from build123d import *

# Parameters (mm, degrees)
SKETCH1_W               = 673.1
SKETCH1_H               = 152.4
BOSS_EXTRUDE1_DEPTH     = 7.9375
SKETCH2_W               = 7.9375
SKETCH2_H               = 123.825
SKETCH2_W_2             = 644.525
SKETCH2_H_2             = 7.9375
BOSS_EXTRUDE2_DEPTH     = 15.875
FILLET1_R               = 6.35
SKETCH3_R               = 9.525
SKETCH3_R_2             = 6.35
CUT_EXTRUDE1_DEPTH      = 1
CUT_EXTRUDE1_DEPTH_BACK = 16.875


with BuildPart() as part:
    # Sketch1 → Boss-Extrude1 (new body, symmetric)
    with BuildSketch(Plane.XY):
        Rectangle(SKETCH1_W, SKETCH1_H)
    extrude(amount=BOSS_EXTRUDE1_DEPTH, both=True)

    # Sketch2 → Boss-Extrude2 (add)
    with BuildSketch(Plane.XY.offset(7.9375)):
        with Locations((-340.51875, 0)):
            Rectangle(SKETCH2_W, SKETCH2_H)
        with Locations((0, 80.16875)):
            Rectangle(SKETCH2_W_2, SKETCH2_H_2)
        with Locations((0, -80.16875)):
            Rectangle(SKETCH2_W_2, SKETCH2_H_2)
        with Locations((340.51875, 0)):
            Rectangle(SKETCH2_W, SKETCH2_H)
    extrude(amount=-BOSS_EXTRUDE2_DEPTH)

    # Fillet1
    fillet1_edges = [part.edges().sort_by_distance(p)[0] for p in [
        (-336.55, -61.9125, 0),
        (-336.55, 61.9125, 0),
        (322.2625, 76.2, 0),
        (-322.2625, 76.2, 0),
        (322.2625, -76.2, 0),
        (-322.2625, -76.2, 0),
        (336.55, 61.9125, 0),
        (336.55, -61.9125, 0),
    ]]
    fillet(fillet1_edges, radius=FILLET1_R)

    # Sketch3 → Cut-Extrude1 (cut, two sides)
    with BuildSketch(Plane.XY.offset(7.9375)) as cut_extrude1_sk:
        with Locations((0, -60.325)):
            Circle(SKETCH3_R)
        with Locations((0, 63.5)):
            Circle(SKETCH3_R_2)
        with Locations((25.4, 63.5)):
            Circle(SKETCH3_R_2)
        with Locations((50.8, 63.5)):
            Circle(SKETCH3_R_2)
        with Locations((76.2, 63.5)):
            Circle(SKETCH3_R_2)
        with Locations((101.6, 63.5)):
            Circle(SKETCH3_R_2)
        with Locations((127, 63.5)):
            Circle(SKETCH3_R_2)
        with Locations((152.4, 63.5)):
            Circle(SKETCH3_R_2)
        with Locations((177.8, 63.5)):
            Circle(SKETCH3_R_2)
        with Locations((203.2, 63.5)):
            Circle(SKETCH3_R_2)
        with Locations((228.6, 63.5)):
            Circle(SKETCH3_R_2)
        with Locations((254, 63.5)):
            Circle(SKETCH3_R_2)
        with Locations((279.4, 63.5)):
            Circle(SKETCH3_R_2)
        with Locations((304.8, 63.5)):
            Circle(SKETCH3_R_2)
        with Locations((-25.4, 63.5)):
            Circle(SKETCH3_R_2)
        with Locations((-50.8, 63.5)):
            Circle(SKETCH3_R_2)
        with Locations((-76.2, 63.5)):
            Circle(SKETCH3_R_2)
        with Locations((-101.6, 63.5)):
            Circle(SKETCH3_R_2)
        with Locations((-127, 63.5)):
            Circle(SKETCH3_R_2)
        with Locations((-152.4, 63.5)):
            Circle(SKETCH3_R_2)
        with Locations((-177.8, 63.5)):
            Circle(SKETCH3_R_2)
        with Locations((-203.2, 63.5)):
            Circle(SKETCH3_R_2)
        with Locations((-228.6, 63.5)):
            Circle(SKETCH3_R_2)
        with Locations((-254, 63.5)):
            Circle(SKETCH3_R_2)
        with Locations((-279.4, 63.5)):
            Circle(SKETCH3_R_2)
        with Locations((-304.8, 63.5)):
            Circle(SKETCH3_R_2)
        with Locations((293.6875, -60.325)):
            Circle(SKETCH3_R)
        with Locations((-293.6875, -60.325)):
            Circle(SKETCH3_R)
    extrude(amount=CUT_EXTRUDE1_DEPTH, mode=Mode.SUBTRACT)
    extrude(cut_extrude1_sk.sketch, amount=-CUT_EXTRUDE1_DEPTH_BACK, mode=Mode.SUBTRACT)


solid = part.part
Source: CAD feature listing. Evaluate the final solid. Frame: model axes, mm. Give positions to 0.01 mm unless a question says otherwise; leave off trailing zeros. Write each loop counter-clockwise with the first axis right and the second up, starting at its lowest first coordinate (ties: lowest second). Pieces come first, ordered by that corner, then holes. Notation, with made-up numbers: M 46,18.25 L 66,18.25 A22 cw 66,48.25 Z; hole C 16,-38.75 d7. An arc over 180 degrees is marked long. Answer as a JSON object with one key per item and string values.
Q1. Ray query, line 1 along X through (y, z) = (-59, -6.5); line 2 along Y through (x, z) = (151.5, -0.75); line 3 along X through (y, z) = (-71, 2.75). Return the intervals inside material, ascending.
Geometry check:
{"line 1": "x = -344.49 to -303.12, -284.26 to -9.43, 9.43 to 284.26, 303.12 to 344.49", "line 2": "y = -84.14 to 57.21, 69.79 to 84.14", "line 3": "x = -336.55 to 336.55"}
Q2. Mould query, pull axis X, two halves, no side actions, for faces 1 (the face through (-26.78, 57.3, 0.11)), 2 (the face through (302.486, -63.973, 0.111)), 3 (the face through (-344.488, -1, 0)), 4 (the face through (-5, 84.138, 0)). Classes: +X half, -X half, draft (parallel to the pull), parting line (faces both ways), or undercut.
Geometry check:
{"face 1": "undercut", "face 2": "undercut", "face 3": "-X half", "face 4": "draft"}
Q3. Cut plane A-A, the plane x = -50.8. Return the cut outline in (y, z), then the cut area to 3 significant figures.
Geometry check:
{"outline": "M -84.14,-7.94 L 57.15,-7.94 L 57.15,7.94 L -84.14,7.94 Z; M 69.85,-7.94 L 84.14,-7.94 L 84.14,7.94 L 69.85,7.94 Z", "area": "2,470 mm^2"}
Q4. Contact query for flat-ended pins moving along their axis: P1, Ø20.5, axis at x = -152.4, y = 63.5, coming from the -Z side; P2, Ø6.5, axis at y = 71.5, z = -4, coming from the -X side; P3, Ø10, axis at x = 177.8, y = 63.5, coming from the -Z side; P4, Ø1.3, axis at y = 83.5, z = -3, coming from the +X side. Output: stop coordinate, or through.
Geometry check:
{"P1": "stops at z = -7.94", "P2": "stops at x = -336.55", "P3": "passes through", "P4": "stops at x = 322.26"}
Q5. Cut plane B-B, the plane z = 0.75. Count the separate pieces of the cut face and the enclosed holes in it, then the cut area to 3 significant figures.
Geometry check:
{"separate pieces": "1", "enclosed holes": "28", "area": "111,000 mm^2"}
